For this review, take the finished solid that the model builds, in its own axes (mm). Face numbers are marked on the shaded views. A direction names the side the tool comes from. Round coordinates to 2 decimals unless told otherwise and drop trailing zeros. Order: outer loops, then holes, each group sorted by start corner. A loop starts at its lowest first (then second) coordinate and runs counter-clockwise, first axis right, second up. Notation, with made-up numbers: (52, 9.5) - (64, 9.5) arc R20 ccw to (64, 25.5) - close; hole circle Ø3 at (4.5, 22.25). An arc over 180 degrees is marked (long way). One line per item, written item: value.
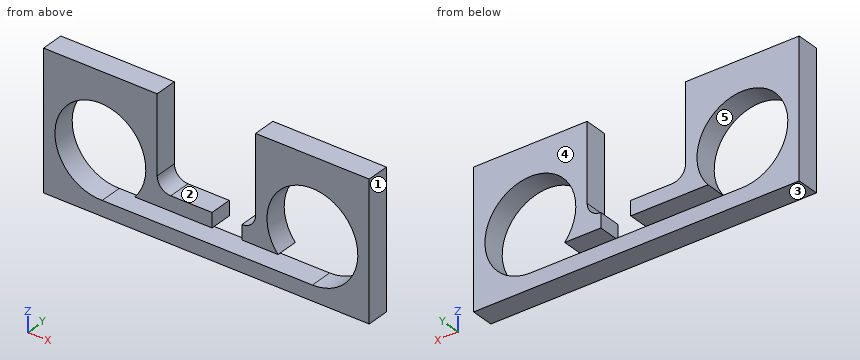
```python
from build123d import *

# Parameters (mm, degrees)
F0_W     = 273.05
F0_H     = 114.3
F1_DEPTH = 19.05
F2_R     = 38.1
F3_DEPTH = 25.4
F5_DEPTH = 25.4
F7_DEPTH = 25.4


with BuildPart() as f1:
    # F0 (on Front) → F1 (new body)
    with BuildSketch(Plane.XZ):
        with Locations((136.525, 57.15)):
            Rectangle(F0_W, F0_H)
    extrude(amount=F1_DEPTH)

    # F2 (on face) → F3 (cut)
    with BuildSketch(Plane.XZ.offset(19.05)):
        with Locations((47.625, 50.8)):
            Circle(F2_R)
        with Locations((225.425, 50.8)):
            Circle(F2_R)
    extrude(amount=-F3_DEPTH, mode=Mode.SUBTRACT)

    # F4 (on face) → F5 (cut)
    with BuildSketch(Plane.XZ.offset(19.05)):
        with BuildLine():
            Line((177.8, 114.3), (95.25, 114.3))
            Line((95.25, 114.3), (95.25, 49.53))
            ThreePointArc((95.25, 49.53), (98.597769, 41.447769), (106.68, 38.1))
            Line((106.68, 38.1), (166.37, 38.1))
            ThreePointArc((166.37, 38.1), (174.452231, 41.447769), (177.8, 49.53))
            Line((177.8, 49.53), (177.8, 114.3))
        make_face()
    extrude(amount=-F5_DEPTH, mode=Mode.SUBTRACT)

    # F6 (on face) → F7 (cut)
    with BuildSketch(Plane.XZ.offset(19.05)):
        Polygon((166.37, 25.869032), (166.37, 38.1), (141.262531, 38.1), (141.262531, 25.869032), (76.435707, 25.869032), (46.121879, 12.729662), (225.418697, 12.700001), (196.614293, 25.869032), align=None)
    extrude(amount=-F7_DEPTH, mode=Mode.SUBTRACT)


solid = f1.part
```
Item 1: Take a section at C-C (y = -9). Write out the cut boundary in (x, z) (3 decimals).
Returned:
outline: (0, 0) - (273.05, 0) - (273.05, 114.3) - (177.8, 114.3) - (177.8, 49.53) arc R11.43 cw to (166.37, 38.1) - (166.37, 25.869) - (196.614, 25.869) arc R38.1 cw (long way) to (225.413, 12.7) - (49.116, 12.729) arc R38.1 cw (long way) to (76.436, 25.869) - (141.263, 25.869) - (141.263, 38.1) - (106.68, 38.1) arc R11.43 cw to (95.25, 49.53) - (95.25, 114.3) - (0, 114.3) - close
Item 2: For P1, Ø1, axis at x = 142.5, y = -5.5, coming from the +Z side; P2, Ø12, axis at x = 188.5, z = 99, coming from the +Y side; P3, Ø9.5, axis at x = 170.5, y = -8, coming from the +Z side; P4, Ø12, axis at x = 29, z = 29, coming from the -Y side, all flat-tipped, find the tip position at first contact; note any pin that passes through.
Returned:
P1: z = 12.71
P2: y = 0
P3: z = 42.33
P4: through
Item 3: Wall thickness on line 1 (X direction, y = -12, z = 50.8) (3 decimals); line 2 (Z direction, x = 125, y = -12.25); line 3 (X direction, y = -7, z = 33.5): over which ranges is each line inside the solid? List them lowest first.
Returned:
line 1: 0 to 9.525, 85.725 to 95.25, 177.8 to 187.325, 263.525 to 273.05
line 2: 0 to 12.72, 25.87 to 38.1
line 3: 0 to 13.68, 81.57 to 141.26, 166.37 to 191.48, 259.37 to 273.05
Item 4: Take a section at A-A (z = 93). Write out the cut boundary in (x, y), plus the area to 3 significant figures.
Returned:
outline: (0, -19.05) - (95.25, -19.05) - (95.25, 0) - (0, 0) - close; (177.8, -19.05) - (273.05, -19.05) - (273.05, 0) - (177.8, 0) - close
area: 3,630 mm^2
Item 5: The part is to be moulded in two halves that separate along Z. For the marked faces 3, 4 and 5, say which applies: +Z half, -Z half, draft (parallel to the pull), parting line (faces both ways), or undercut.
Returned:
face 3: -Z half
face 4: draft
face 5: undercut
Item 6: Machinability: for the marked faces 1 and 2, which of the approach directions +Z, -Z, +X, -X, +Y, -Y give a long, thin tool a straight path to every point of the face, cutting with its end or side? Answer none if there is none.
Returned:
face 1: +Z, -Z, +X, +Y, -Y
face 2: +Z, +Y, -Y
Item 7: Take a section at B-B (x = 74). Write out the cut boundary in (y, z).
Returned:
outline: (-19.05, 0) - (0, 0) - (0, 12.73) - (-19.05, 12.73) - close; (-19.05, 78.29) - (0, 78.29) - (0, 114.3) - (-19.05, 114.3) - close
Item 8: Take a section at D-D (z = 67). Write out the cut boundary in (x, y).
Returned:
outline: (0, -19.05) - (13.14, -19.05) - (13.14, 0) - (0, 0) - close; (82.11, -19.05) - (95.25, -19.05) - (95.25, 0) - (82.11, 0) - close; (177.8, -19.05) - (190.94, -19.05) - (190.94, 0) - (177.8, 0) - close; (259.91, -19.05) - (273.05, -19.05) - (273.05, 0) - (259.91, 0) - close
